Input: part model. Units: mm. Frame: model coordinates. A direction names the side the tool comes from. Round coordinates to 2 decimals unless told otherwise and drop trailing zeros. Order: outer loops, then holes, each group sorted by start corner. A loop starts at its lowest first (then second) coordinate and runs counter-clockwise, first axis right, second up. Notation, with made-up numbers: (36.5, -18) -> (51.5, -18) arc R20 ccw to (51.5, 16) -> close; hole circle Ø11 at (60, -26.5). An arc over 180 degrees is marked (long way). Use a Markdown table: item, result.
from build123d import *

# Parameters (mm, degrees)
F0_W     = 24
F0_H     = 34.397194515
F1_DEPTH = 25
F2_W     = 3
F2_H     = 34.397194515
F3_DEPTH = 4.7
F4_T     = -0.61


with BuildPart() as f1:
    # F0 (on Front) → F1 (new body)
    with BuildSketch(Plane.XZ):
        with Locations((12, 17.1985972575)):
            Rectangle(F0_W, F0_H)
    extrude(amount=F1_DEPTH)

    # F2 (on face) → F3 (cut)
    with BuildSketch(Plane.XZ.offset(25)):
        with Locations((10.9055030495, 17.1985972575)):
            Rectangle(F2_W, F2_H)
    extrude(amount=-F3_DEPTH, mode=Mode.SUBTRACT)

    # F4
    f4_openings = [f1.faces().sort_by_distance(p)[0] for p in [
        (12, 0, 17.198597),
        (0, -12.5, 17.198597),
        (12.02634, -12.255735, 0),
        (24, -12.5, 17.198597),
        (12.02634, -12.255735, 34.397195),
    ]]
    offset(amount=F4_T, openings=f4_openings, kind=Kind.INTERSECTION)


solid = f1.part
1) Set-up query: faces 1 (the face through (18, -25, 17)), 2 (the face through (11, -20.3, 17)), 3 (the face through (4, -24.39, 17)). Return all of +Z, -Z, +X, -X, +Y, -Y with unobstructed straight access to the full face (end or side cutting, diameter ignored); none if empty.
Answer key:
| item | result |
|---|---|
| face 1 | +Z, -Z, +X, -X, -Y |
| face 2 | +Z, -Z, -Y |
| face 3 | +Z, -Z, -X, +Y |
2) Contact query for flat-ended pins moving along their axis: P1, Ø5.5, axis at x = 18.5, z = 11, coming from the +Y side; P2, Ø3.5, axis at x = 11.5, z = 17, coming from the -Y side; P3, Ø2, axis at y = -22, z = 29, coming from the -X side. Output: stop coordinate, or through.
Answer key:
| item | result |
|---|---|
| P1 | stops at y = -24.39 |
| P2 | stops at y = -25 |
| P3 | stops at x = 8.8 |
3) Ray query, probe 1 along X at (y, z) = (-23.75, 21); probe 2 along Y at (x, z) = (8, 5.5); probe 3 along X at (y, z) = (-20, 27). Return the intervals inside material, ascending.
Answer key:
| item | result |
|---|---|
| probe 1 | x = 8.8 to 9.41, 12.41 to 13.02 |
| probe 2 | y = -25 to -24.39 |
| probe 3 | x = 8.8 to 13.02 |
4) Cut plane A-A on y = -21.1. Return loops of the section in (x, z), and give its area (3 significant figures).
Answer key:
| item | result |
|---|---|
| outline | (8.8, 0) -> (9.41, 0) -> (9.41, 34.4) -> (8.8, 34.4) -> close; (12.41, 0) -> (13.02, 0) -> (13.02, 34.4) -> (12.41, 34.4) -> close |
| area | 42.0 mm^2 |
5) Cut plane B-B on z = 23.5. Return loops of the section in (x, y), and give its area (3 significant figures).
Answer key:
| item | result |
|---|---|
| outline | (0, -25) -> (9.41, -25) -> (9.41, -20.3) -> (12.41, -20.3) -> (12.41, -25) -> (24, -25) -> (24, -24.39) -> (13.02, -24.39) -> (13.02, -19.69) -> (8.8, -19.69) -> (8.8, -24.39) -> (0, -24.39) -> close |
| area | 20.4 mm^2 |
6) Draft query along X for faces 4 (the face through (12.406, -23, 17)), 5 (the face through (18, -24.39, 17)), 6 (the face through (13.016, -22, 17)). Return one class per face: released by +X, released by -X, zero draft, split by the parting line, or undercut.
Answer key:
| item | result |
|---|---|
| face 4 | undercut |
| face 5 | zero draft |
| face 6 | released by +X |
7) Cut plane C-C on x = 10.5. Return loops of the section in (y, z).
Answer key:
| item | result |
|---|---|
| outline | (-20.3, 0) -> (-19.69, 0) -> (-19.69, 34.4) -> (-20.3, 34.4) -> close |
